from build123d import *

# Parameters (mm, degrees)
CROQUIS1_R              = 4.35
SALIENTE_EXTRUIR1_DEPTH = 14.7
CROQUIS2_R              = 4.35
CORTAR_EXTRUIR1_DEPTH   = 2.2


with BuildPart() as part:
    # Croquis1 → Saliente-Extruir1 (new body)
    with BuildSketch(Plane(origin=(0, 0, 0), x_dir=(0, 0, -1), z_dir=(1, 0, 0))):
        with BuildLine():
            Line((19.366750419, 5), (-19.366750419, 5))
            ThreePointArc((-19.366750419, 5), (-20.810126092, 5.212864461), (-22.130604411, 5.833333333))
            ThreePointArc((-22.130604411, 5.833333333), (-33, 0), (-22.130604411, -5.833333333))
            ThreePointArc((-22.130604411, -5.833333333), (-20.810126092, -5.212864461), (-19.366750419, -5))
            Line((-19.366750419, -5), (19.366750419, -5))
            ThreePointArc((19.366750419, -5), (20.810126092, -5.212864461), (22.130604411, -5.833333333))
            ThreePointArc((22.130604411, -5.833333333), (33, 0), (22.130604411, 5.833333333))
            ThreePointArc((22.130604411, 5.833333333), (20.810126092, 5.212864461), (19.366750419, 5))
        make_face()
        with Locations((-26, 0)):
            Circle(CROQUIS1_R, mode=Mode.SUBTRACT)
        with Locations((26, 0)):
            Circle(CROQUIS1_R, mode=Mode.SUBTRACT)
    extrude(amount=SALIENTE_EXTRUIR1_DEPTH)

    # Croquis2 → Cortar-Extruir1 (cut)
    with BuildSketch(Plane(origin=(14.7, 0, 0), x_dir=(0, 0, -1), z_dir=(1, 0, 0))):
        with BuildLine():
            Line((-17.5, 0), (-14.5, 5))
            Line((-14.5, 5), (-19.366750419, 5))
            ThreePointArc((-19.366750419, 5), (-20.810126092, 5.212864461), (-22.130604411, 5.833333333))
            ThreePointArc((-22.130604411, 5.833333333), (-33, 0), (-22.130604411, -5.833333333))
            ThreePointArc((-22.130604411, -5.833333333), (-20.810126092, -5.212864461), (-19.366750419, -5))
            Line((-19.366750419, -5), (-14.5, -5))
            Line((-14.5, -5), (-17.5, 0))
        make_face()
        with Locations((-26, 0)):
            Circle(CROQUIS2_R, mode=Mode.SUBTRACT)
    extrude(amount=-CORTAR_EXTRUIR1_DEPTH, mode=Mode.SUBTRACT)


solid = part.part
Work out the finished part from the listing and answer in its coordinate system (mm). A direction names the side the tool comes from. Round coordinates to 2 decimals unless told otherwise and drop trailing zeros. Loops run counter-clockwise (first coordinate to the right, second up) from the corner with the lowest first, then second, coordinate; pieces in that order, holes last. Notation, with made-up numbers: (81.5, 62) - (125.5, 62) arc R8 ccw to (125.5, 75) - close; hole circle Ø6 at (-30.5, -29). An arc over 180 degrees is marked (long way). One line per item, written item: value.
Q1. Find section D-D on z = 26. Give the vertices of the cut face in (x, y), and give its area (4 significant figures).
Check values:
outline: (0, -7) - (12.5, -7) - (12.5, -4.35) - (0, -4.35) - close; (0, 4.35) - (12.5, 4.35) - (12.5, 7) - (0, 7) - close
area: 66.25 mm2
Q2. For faces 1 (the cylindrical face through (7.247, -5.207, -20.79)), 2 (the flat face through (13.6, 2.5, 16)), 3 (the cylindrical face through (6.162, 5.207, 20.79)), determine the directions among +Z, -Z, +X, -X, +Y, -Y from which every point of the face is accessible in a straight line to the end or side of a thin tool.
Check values:
face 1: +X, -X, -Y
face 2: +Z, +X, +Y
face 3: +X, -X, +Y
Q3. The mould has two halves that part along Z. Classify faces 4 (the flat face through (13.6, -2.5, 16)), 5 (the cylindrical face through (7.25, 5.22, -20.83)), 6 (the flat face through (14.7, 0, -7)): +Z half, -Z half, draft (parallel to the pull), parting line (faces both ways), or undercut.
Check values:
face 4: +Z half
face 5: undercut
face 6: draft
Q4. Find section A-A on z = -26. Give the vertices of the cut face in (x, y).
Check values:
outline: (0, -7) - (14.7, -7) - (14.7, -4.35) - (0, -4.35) - close; (0, 4.35) - (14.7, 4.35) - (14.7, 7) - (0, 7) - close
Q5. Find section B-B on x = 10.5. Give the vertices of the cut face in (y, z), and give its area (3 significant figures).
Check values:
outline: (-5.83, -22.13) arc R7 ccw (long way) to (5.83, -22.13) arc R5 cw to (5, -19.37) - (5, 19.37) arc R5 cw to (5.83, 22.13) arc R7 ccw (long way) to (-5.83, 22.13) arc R5 cw to (-5, 19.37) - (-5, -19.37) arc R5 cw to start; hole circle Ø8.7 at (0, -26); hole circle Ø8.7 at (0, 26)
area: 583 mm2
Q6. Each of these flat-tipped pins is pushed along its axis until it touches: pin 1 Ø6 at (x, y) = (13, -4.5) entering from -Z; pin 2 Ø1 at (x, y) = (4, -5) entering from +Z; pin 3 Ø7.5 at (x, z) = (6.5, -8) entering from -Y. Where does it stop, or does it pass through?
Check values:
pin 1: z = -32.84
pin 2: z = 31.36
pin 3: y = -5
Q7. Straight lines are drawn through the part: probe 1 along Y at (x, z) = (6.25, 26); probe 2 along Z at (x, y) = (9.5, -1.75); probe 3 along Z at (x, y) = (9.5, 1.25). For each, find the intervals that lie inside material, in ascending order.
Check values:
probe 1: -7 to -4.35, 4.35 to 7
probe 2: -32.78 to -29.98, -22.02 to 22.02, 29.98 to 32.78
probe 3: -32.89 to -30.17, -21.83 to 21.83, 30.17 to 32.89
Q8. Find section C-C on y = -3.5. Give the vertices of the cut face in (x, z).
Check values:
outline: (0, -32.06) - (14.7, -32.06) - (14.7, -28.58) - (0, -28.58) - close; (0, -23.42) - (14.7, -23.42) - (14.7, 15.4) - (12.5, 15.4) - (12.5, 23.42) - (0, 23.42) - close; (0, 28.58) - (12.5, 28.58) - (12.5, 32.06) - (0, 32.06) - close
